Here's the drawing with two shaded views (mm, measured from the low corner). I have some questions. A direction names the side the tool comes from. Round coordinates to 2 decimals unless told otherwise and drop trailing zeros. Loops run counter-clockwise (first coordinate to the right, second up) from the corner with the lowest first, then second, coordinate; pieces in that order, holes last. Notation, with made-up numbers: M 4.5,-25 L 47.5,-25 A24 ccw 47.5,-8 Z; hole C -20.75,-31.5 d2. An arc over 180 degrees is marked long. Answer as CSV lines item,"result".
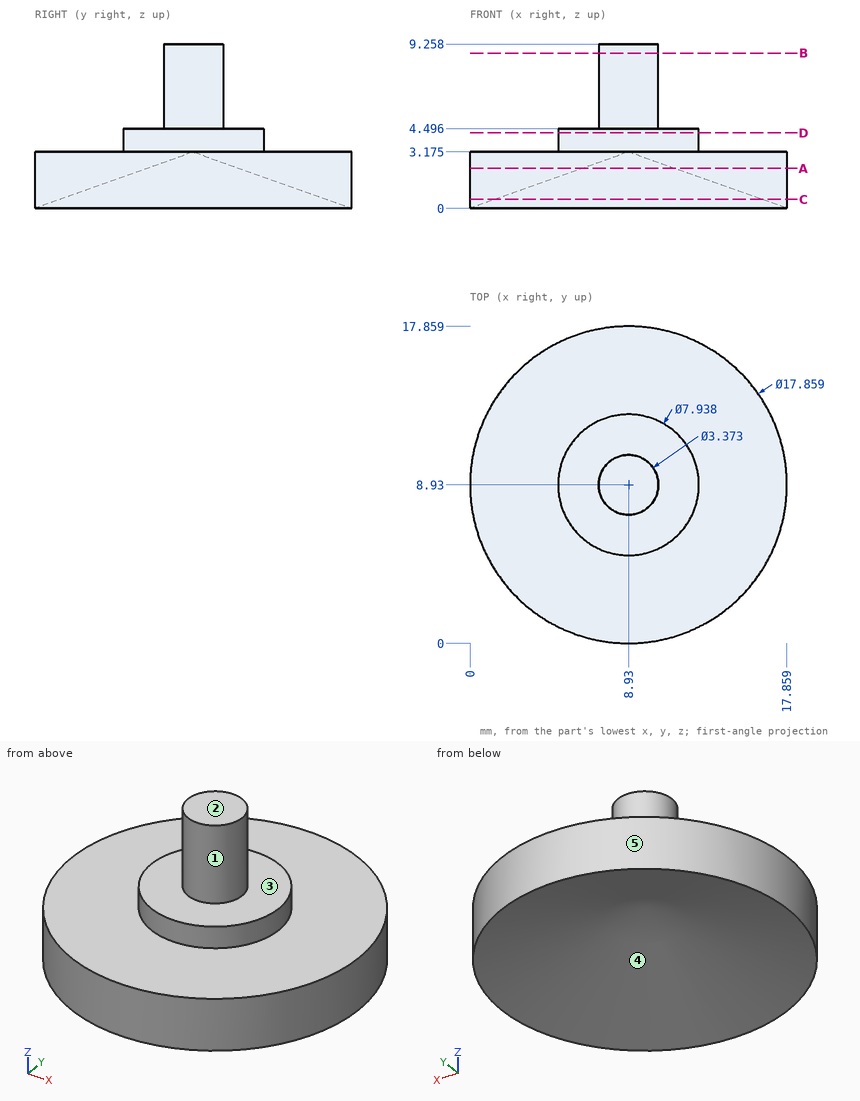
1. I want a section at A-A, the plane z = 2.25. Please give me the cut outline in (x, y), and give its area (3 significant figures).
Evaluation:
outline,"C 8.93,8.93 d17.86; hole C 8.93,8.93 d5.2"
area,"229 mm²"
2. I want a section at B-B, the plane z = 8.75. Please give me the cut outline in (x, y).
Evaluation:
outline,"C 8.93,8.93 d3.37"
3. We'd pull the mould along X, two halves only. Please class the marked faces 3, 4 and 5: pulls with the +X half, pulls with the -X half, needs draft (parallel to the pull), parting line crosses it, or undercut.
Evaluation:
face 3,"needs draft"
face 4,"undercut"
face 5,"parting line crosses it"
4. If I drill on line 1 (Z direction, x = 13.75, y = 1.75) (1 decimal); line 2 (Z direction, x = 10.25, y = 1.25) (1 decimal); line 3 (X direction, y = 16.25, z = 1.25) (1 decimal), over which ranges is the centre line in solid material (lowest first)? Write a range as [from, to].
Evaluation:
line 1,"z = [0.1, 3.2]"
line 2,"z = [0.4, 3.2]"
line 3,"x = [3.8, 14]"
5. I want a section at C-C, the plane z = 0.5. Please give me the cut outline in (x, y).
Evaluation:
outline,"C 8.93,8.93 d17.86; hole C 8.93,8.93 d15.05"
6. For P1, Ø1, axis at x = 5.5, z = 4, coming from the -Y side; P2, Ø4, axis at y = 12, z = 1, coming from the -X side (1 decimal); P3, Ø6, axis at x = 4, y = 9, coming from the +Z side, each with a flat end and sliding along its axis, tell me the tip position at first contact or that it passes through.
Evaluation:
P1,"stops at y = 6.25"
P2,"stops at x = 0.1"
P3,"stops at z = 4.5"
7. Which directions (+Z, -Z, +X, -X, +Y, -Y) give clear straight access to the entire face, cutting with the end or side of a thin tool? Please do the marked faces 1 and 2.
Evaluation:
face 1,"+Z"
face 2,"+Z, +X, -X, +Y, -Y"
8. I want a section at D-D, the plane z = 4.25. Please give me the cut outline in (x, y).
Evaluation:
outline,"C 8.93,8.93 d7.94"
